```python
from build123d import *

# Parameters (mm, degrees)
SKETCH_1_R      = 3.5
SKETCH_1_R_2    = 3
EXTRUDE_1_DEPTH = 2


with BuildPart() as part:
    # Sketch 1 → Extrude 1 (new, symmetric)
    with BuildSketch(Plane.XY):
        with BuildLine():
            ThreePointArc((-3.844739387, -1.103620878), (-2.213352607, -9.345380488), (-1.984991162, -17.743944374))
            Line((-1.984991162, -17.743944374), (-4.492709151, -61.743944374))
            ThreePointArc((-4.492709151, -61.743944374), (0, -66.5), (4.492709151, -61.743944374))
            Line((4.492709151, -61.743944374), (1.984991162, -17.743944374))
            ThreePointArc((1.984991162, -17.743944374), (2.213352607, -9.345380488), (3.844739387, -1.103620878))
            ThreePointArc((3.844739387, -1.103620878), (0, 4), (-3.844739387, -1.103620878))
        make_face()
        with Locations((0, -62)):
            Circle(SKETCH_1_R, mode=Mode.SUBTRACT)
        Circle(SKETCH_1_R_2, mode=Mode.SUBTRACT)
    extrude(amount=EXTRUDE_1_DEPTH, both=True)


solid = part.part
```
Verification items for the finished model (mm, model axes). A direction names the side the tool comes from. Round coordinates to 2 decimals unless told otherwise and drop trailing zeros. Order: outer loops, then holes, each group sorted by start corner. A loop starts at its lowest first (then second) coordinate and runs counter-clockwise, first axis right, second up. Notation, with made-up numbers: (-37.75, 89.25) -> (17.25, 89.25) arc R16 cw to (17.25, 111.25) -> close; hole circle Ø1 at (-28.5, -22.75). An arc over 180 degrees is marked (long way). Put each result on its own line as item: value. Start each with the question number.
(1) Section check C-C (z = 0.4). Enter the section's corners in (x, y) (3 decimals).
(2) Material ranges on line 1 along Y through (x, z) = (-0.25, 1.8); line 2 along X through (y, z) = (-14, 1.45); line 3 along X through (y, z) = (-59, -1.65), recorded low to high.
(3) Section check A-A (x = 0). Enter the section's corners in (y, z), then the cut area to 3 significant figures.
(4) Draft check along Y on faces 1 (the face through (-3, 0, 0)), 2 (the face through (0, -31, 2)), 3 (the face through (-3.22, -39.44, 0.03)). Enter one of: +Y half, -Y half, draft (parallel to the pull), parting line (faces both ways), or undercut.
(5) Depth check by flat-ended pin: pin 1 Ø1.5 at (y, z) = (-20.5, -1.5) entering from +X; pin 2 Ø1 at (x, z) = (1.5, -0.5) entering from -Y. Enter the tip coordinate at first touch or a pass-through.
(6) Tool access check on faces 4 (the face through (0, 4, 0)), 5 (the face through (3.256, -40.052, 0.028)). Record the directions out of +Z, -Z, +X, -X, +Y, -Y that give a thin tool (end or side, any length) a straight path to the whole face; none if there is none.
(7) Section check D-D (y = -11). Enter the section's corners in (x, z), then the cut area to 3 significant figures.
(8) Section check B-B (y = 0). Enter the section's corners in (x, z).
Completed:
1. outline: (-4.493, -61.744) arc R4.5 ccw (long way) to (4.493, -61.744) -> (1.985, -17.744) arc R50 cw to (3.845, -1.104) arc R4 ccw (long way) to (-3.845, -1.104) arc R50 cw to (-1.985, -17.744) -> close; hole circle Ø7 at (0, -62); hole circle Ø6 at (0, 0)
2. line 1: y = -66.49 to -65.49, -58.51 to -2.99, 2.99 to 3.99
2. line 2: x = -1.91 to 1.91
2. line 3: x = -4.34 to -1.8, 1.8 to 4.34
3. outline: (-66.5, -2) -> (-65.5, -2) -> (-65.5, 2) -> (-66.5, 2) -> close; (-58.5, -2) -> (-3, -2) -> (-3, 2) -> (-58.5, 2) -> close; (3, -2) -> (4, -2) -> (4, 2) -> (3, 2) -> close
3. area: 230 mm2
4. face 1: undercut
4. face 2: draft
4. face 3: undercut
5. pin 1: stops at x = 2.18
5. pin 2: stops at y = -66.39
6. face 4: +Z, -Z
6. face 5: +Z, -Z, +X
7. outline: (-2.06, -2) -> (2.06, -2) -> (2.06, 2) -> (-2.06, 2) -> close
7. area: 16.4 mm2
8. outline: (-4, -2) -> (-3, -2) -> (-3, 2) -> (-4, 2) -> close; (3, -2) -> (4, -2) -> (4, 2) -> (3, 2) -> close
